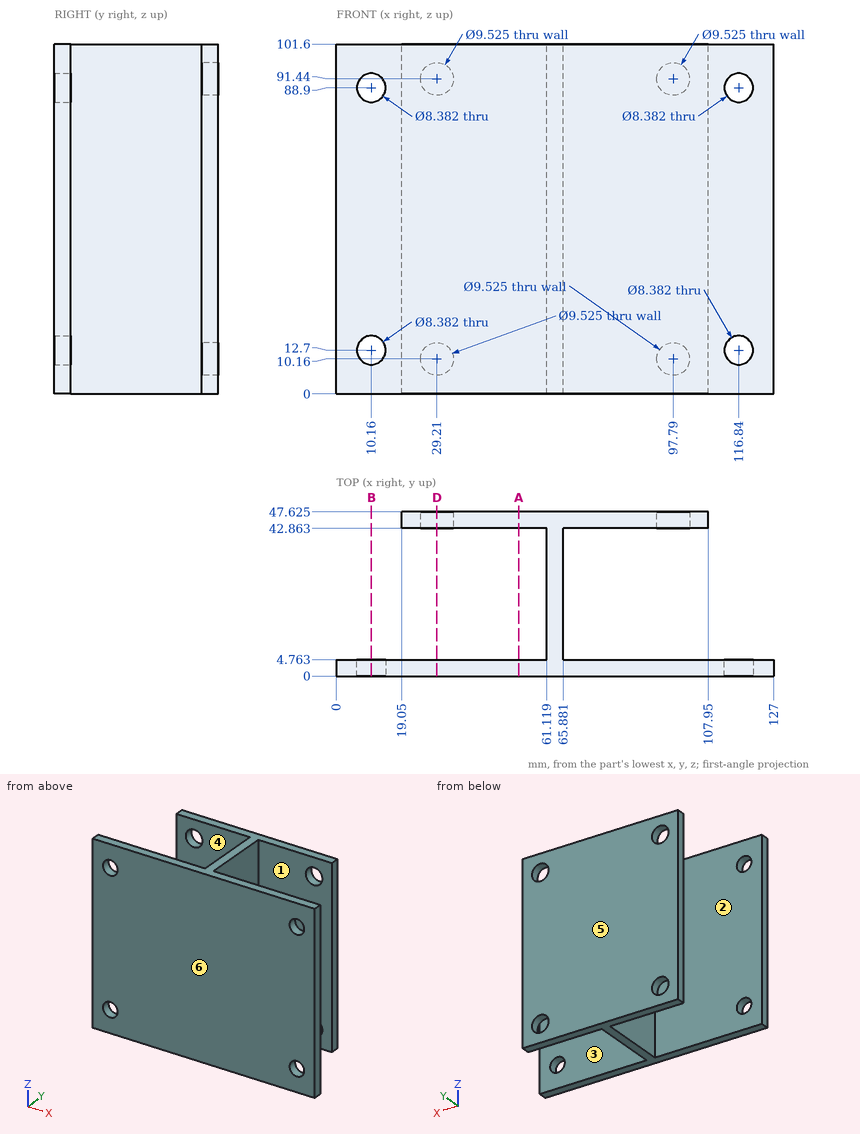
Design review of the part shown in the three views and the two pictorial views. Dimensions are in mm from the part's minimum x, y and z. A direction names the side the tool comes from. Round coordinates to 2 decimals unless told otherwise and drop trailing zeros. Write each loop counter-clockwise with the first axis right and the second up, starting at its lowest first coordinate (ties: lowest second). Pieces come first, ordered by that corner, then holes.
1) Take a section at A-A on x = 53. Give the boundary of the cut face in (y, z) (1 decimal).
Answer below:
outline: (0, 0) - (4.8, 0) - (4.8, 101.6) - (0, 101.6) - close; (42.9, 0) - (47.6, 0) - (47.6, 101.6) - (42.9, 101.6) - close
2) Machinability: for the marked faces 1 and 2, which of the approach directions +Z, -Z, +X, -X, +Y, -Y give a long, thin tool a straight path to every point of the face, cutting with its end or side? Answer none if there is none.
Answer below:
face 1: +Z, -Z, +X
face 2: +Z, -Z, -X
3) Take a section at D-D on x = 29.21. Give the boundary of the cut face in (y, z) (1 decimal), then the cut area to 3 significant figures.
Answer below:
outline: (0, 0) - (4.8, 0) - (4.8, 101.6) - (0, 101.6) - close; (42.9, 0) - (47.6, 0) - (47.6, 5.4) - (42.9, 5.4) - close; (42.9, 14.9) - (47.6, 14.9) - (47.6, 86.7) - (42.9, 86.7) - close; (42.9, 96.2) - (47.6, 96.2) - (47.6, 101.6) - (42.9, 101.6) - close
area: 877 mm2
4) For line 1 along Z through (x, y) = (10.16, 1.95); line 2 along Z through (x, y) = (29, 45); line 3 along Y through (x, z) = (86, 86) (1 decimal), list the stretches that pass through material, from the lowest coordinate up.
Answer below:
line 1: z = 0 to 8.51, 16.89 to 84.71, 93.09 to 101.6
line 2: z = 0 to 5.4, 14.92 to 86.68, 96.2 to 101.6
line 3: y = 0 to 4.8, 42.9 to 47.6
5) Take a section at B-B on x = 10.16. Give the boundary of the cut face in (y, z).
Answer below:
outline: (0, 0) - (4.76, 0) - (4.76, 8.51) - (0, 8.51) - close; (0, 16.89) - (4.76, 16.89) - (4.76, 84.71) - (0, 84.71) - close; (0, 93.09) - (4.76, 93.09) - (4.76, 101.6) - (0, 101.6) - close
6) Insertion check: pin 1 Ø11 at (x, z) = (116.84, 12.7) entering from +Y; pin 2 Ø4 at (y, z) = (10.5, 83.5) entering from +X; pin 3 Ø2.5 at (y, z) = (44, 55.5) entering from +X. Each pin has a flat end and moves straight along its axis. Give the tip position at first contact, or say it passes through.
Answer below:
pin 1: stops at y = 4.76
pin 2: stops at x = 65.88
pin 3: stops at x = 107.95
7) Mouldability with a two-part tool opening along Y and no side actions: class the marked faces 3, 4, 5 and 6 as +Y half, -Y half, draft (parallel to the pull), parting line (faces both ways), or undercut.
Answer below:
face 3: undercut
face 4: undercut
face 5: +Y half
face 6: -Y half
